Autodesk Inventor part; units mm, degrees
ref_plane "YZ Plane" through (0, 0, 0) normal (1, 0, 0) x (0, 1, 0)
ref_plane "XZ Plane" through (0, 0, 0) normal (0, 1, 0) x (-1, 0, 0)
ref_plane "XY Plane" through (0, 0, 0) normal (0, 0, 1) x (1, 0, 0)
sketch "Sketch1" plane through (0, 0, 0) normal (1, 0, 0) x (0, 1, 0)
  point P0 (0, 0)
sketch "Sketch2" plane through (0, 0, 0) normal (0, 0, 1) x (1, 0, 0)
  circle A0 centre (0, 0) radius 11.5
  line L0 (0, 0) -> (16.9235, 17.0175)
  circle A1 centre (16.9235, 17.0175) radius 4
  circle A2 centre (16.9235, 17.0175) radius 7
  circle A3 centre (-17.0175, 16.9235) radius 4
  circle A4 centre (-17.0175, 16.9235) radius 7
  circle A5 centre (-16.9235, -17.0175) radius 4
  circle A6 centre (-16.9235, -17.0175) radius 7
  circle A7 centre (17.0175, -16.9235) radius 4
  circle A8 centre (17.0175, -16.9235) radius 7
  line L1 (0, 0) -> (54, 0)
  circle A9 centre (54, 0) radius 7.5
  circle A10 centre (54, 0) radius 13
  line L2 (34.0355, 0) -> (34.0355, 8)
  line L3 (34.0355, 8) -> (34.0355, -8)
  line L4 (34.0355, -8) -> (43.753, -8)
  line L5 (23.6854, -8) -> (34.0355, -8)
  line L6 (34.0355, 8) -> (43.753, 8)
  line L7 (34.0355, 8) -> (23.6854, 8)
  arc A11 (-19.5919, 13.8621) -> (-21.1769, 11.2933) centre (0, 0) ccw
  arc A12 (11.96, 21.9535) -> (-12.0815, 21.8869) centre (0, 0) ccw
  arc A13 (-21.9535, 11.96) -> (-21.8869, -12.0815) centre (0, 0) ccw
  arc A14 (-11.96, -21.9535) -> (12.0815, -21.8869) centre (0, 0) ccw
  arc A15 (21.9535, -11.96) -> (21.8869, 12.0815) centre (0, 0) ccw
  dimension "d1" = 23
  dimension "d4" = 8
  dimension "d5" = 14
  dimension "d8" = 360
  dimension "d10" = 54
  dimension "d11" = 15
  dimension "d12" = 26
  dimension "d13" = 8
  dimension "d14" = 16
extrude "Extrusion1" add sketch "Sketch2" along normal blind 10 contours L1 A15 A8 A14 A6 A13 A4 A12 A2 L0 A0 | A0 L0 A2 A15 L1 | A15 L7 L2 L1 | L1 L3 L5 A15 | A2 | L2 L6 A10 L1 | L1 A10 L4 L3 | A10 | A8 | A4 | A6 | A9
extrude "Extrusion2" cut sketch "Sketch2" along normal blind 10 contours A9
fillet "Fillet1" radius 4 2 edges at (23.6854, -8, 5) (21.9535, -11.96, 5)
fillet "Fillet2" radius 6 6 edges at (11.96, 21.9535, 5) (-12.0815, 21.8869, 5) (-21.9535, 11.96, 5) (-21.8869, -12.0815, 5) (-11.96, -21.9535, 5) (12.0815, -21.8869, 5)
properties part number "hw13"
Part model, mm, in its own coordinate system. A direction names the side the tool comes from. Round coordinates to 2 decimals unless told otherwise and drop trailing zeros. Order: outer loops, then holes, each group sorted by start corner. A loop starts at its lowest first (then second) coordinate and runs counter-clockwise, first axis right, second up. Notation, with made-up numbers: M 10.5,72 L 32.5,72 A17 ccw 32.5,86 Z; hole C 88,82 d1. An arc over 180 degrees is marked long. Put each result on its own line as item: value. Start each with the question number.
1. Drop flat-ended pins along their axis: pin 1 (1.5 mm diameter, centred on x = 52, z = 7, fed in from -Y); pin 2 (4 mm diameter, centred on x = 50, z = 7, fed in from -Y); pin 3 (4 mm diameter, centred on y = 14.5, z = 2.5, fed in from -X). Give the stop position or say it passes through.
2. Tool access for faces 4 (the face through (22.865, 10.11, 4.93)), 5 (the face through (-25, 0, 5)): list every direction of +Z, -Z, +X, -X, +Y, -Y with a clear straight run to the whole face (end or side of a thin tool).
3. Drill centre lines: probe 1 along X at (y, z) = (0, 2.5); probe 2 along Y at (x, z) = (0.5, 5.5); probe 3 along X at (y, z) = (-16, 4). Where is each one in solid material? Low to high. Write a range as [from, to].
4. Slice it at C-C on x = -15. List the corners of the cut face in (y, z).
5. Slice it at B-B on x = 0. List the corners of the cut face in (y, z), then the cut area to 3 significant figures.
6. Slice it at D-D on x = 54. List the corners of the cut face in (y, z).
7. Two-plate mould, pull along Y, no slides. Class faces 1 (the face through (35, -8, 5)), 2 (the face through (67, 0, 5)), 3 (the face through (-15.078, -13.469, 4.93)): +Y half, -Y half, draft (parallel to the pull), parting line (faces both ways), or undercut.
8. Slice it at A-A on y = 0. List the corners of the cut face in (x, z).
Findings:
1. pin 1: y = -12.94
1. pin 2: y = -12.85
1. pin 3: x = -24
2. face 4: +Z, -Z
2. face 5: +Z, -Z, -X
3. probe 1: [-25, -11.5], [11.5, 46.5], [61.5, 67]
3. probe 2: [-24.99, -11.49], [11.49, 24.99]
3. probe 3: [-23.85, -20.79], [-13.06, 13.13], [20.91, 23.96]
4. outline: M -23.75,0 L -20.52,0 L -20.52,10 L -23.75,10 Z; M -13.51,0 L 13.47,0 L 13.47,10 L -13.51,10 Z; M 20.38,0 L 23.63,0 L 23.63,10 L 20.38,10 Z
5. outline: M -25,0 L -11.5,0 L -11.5,10 L -25,10 Z; M 11.5,0 L 25,0 L 25,10 L 11.5,10 Z
5. area: 270 mm2
6. outline: M -13,0 L -7.5,0 L -7.5,10 L -13,10 Z; M 7.5,0 L 13,0 L 13,10 L 7.5,10 Z
7. face 1: -Y half
7. face 2: parting line
7. face 3: undercut
8. outline: M -25,0 L -11.5,0 L -11.5,10 L -25,10 Z; M 11.5,0 L 46.5,0 L 46.5,10 L 11.5,10 Z; M 61.5,0 L 67,0 L 67,10 L 61.5,10 Z
